from build123d import *

# Parameters (mm, degrees)
SKETCH2_R           = 19.5
SKETCH2_R_2         = 14.5
BOSS_EXTRUDE1_DEPTH = 20
BOSS_EXTRUDE2_START = 2
SKETCH3_R           = 19.5
BOSS_EXTRUDE2_DEPTH = 2
SKETCH4_R           = 2.85
BOSS_EXTRUDE3_DEPTH = 6


with BuildPart() as part:
    # Sketch2 → Boss-Extrude1 (new body)
    with BuildSketch(Plane(origin=(0, 0, 0), x_dir=(1, 0, 0), z_dir=(0, 1, 0))):
        with Locations(Location((0, 0, 0), (0, 0, 270))):
            Circle(SKETCH2_R)
        with Locations(Location((0, 0, 0), (0, 0, 270))):
            Circle(SKETCH2_R_2, mode=Mode.SUBTRACT)
    extrude(amount=BOSS_EXTRUDE1_DEPTH)

    # Sketch3 → Boss-Extrude2 (add)
    with BuildSketch(Plane.XZ.offset(BOSS_EXTRUDE2_START)):
        with Locations(Location((0, 0, 0), (0, 0, 270))):
            Circle(SKETCH3_R)
    extrude(amount=-BOSS_EXTRUDE2_DEPTH)

    # Sketch4 → Boss-Extrude3 (add)
    with BuildSketch(Plane.XZ.offset(2)):
        with Locations(Location((0, 0, 0), (0, 0, 270))):
            Circle(SKETCH4_R)
    extrude(amount=BOSS_EXTRUDE3_DEPTH)


solid = part.part
Check sheet for the modelled part. Datum: model origin and axes. Units: mm. A direction names the side the tool comes from. Coordinates: 2 decimals unless noted, no trailing zeros. Write each loop counter-clockwise with the first axis right and the second up, starting at its lowest first coordinate (ties: lowest second). Pieces come first, ordered by that corner, then holes. Notation, with made-up numbers: M 24,-25.5 L 53,-25.5 A19 cw 53,7.5 Z; hole C 26,-5.75 d7. An arc over 180 degrees is marked long. Answer as CSV lines item,"result".
Q1. Cross-section at C-C (y = 7.5). Record the boundary of the cut face in (x, z), then the cut area to 3 significant figures.
Check result:
outline,"C 0,0 d39; hole C 0,0 d29"
area,"534 mm^2"
Q2. Mould release check, pull along X, two halves, no side actions. Record for faces 1 (the face through (0, 0, 0)), 2 (the face through (-4, -2, 0)), 3 (the face through (-1.734, -4.958, 2.262)): released by +X, released by -X, zero draft, split by the parting line, or undercut.
Check result:
face 1,"undercut"
face 2,"zero draft"
face 3,"split by the parting line"
Q3. Material ranges on probe 1 along X at (y, z) = (12.5, 0); probe 2 along Y at (x, z) = (9, -14.5); probe 3 along X at (y, z) = (7.5, 2), recorded low to high. Write a range as from..to.
Check result:
probe 1,"-19.5..-14.5, 14.5..19.5"
probe 2,"-2..20"
probe 3,"-19.4..-14.36, 14.36..19.4"
Q4. Cross-section at B-B (x = -2). Record the boundary of the cut face in (y, z), then the cut area to 3 significant figures.
Check result:
outline,"M -8,-2.03 L -2,-2.03 L -2,-19.4 L 20,-19.4 L 20,-14.36 L 0,-14.36 L 0,14.36 L 20,14.36 L 20,19.4 L -2,19.4 L -2,2.03 L -8,2.03 Z"
area,"303 mm^2"
Q5. Cross-section at A-A (z = 0). Record the boundary of the cut face in (x, y), then the cut area to 3 significant figures.
Check result:
outline,"M -19.5,-2 L -2.85,-2 L -2.85,-8 L 2.85,-8 L 2.85,-2 L 19.5,-2 L 19.5,20 L 14.5,20 L 14.5,0 L -14.5,0 L -14.5,20 L -19.5,20 Z"
area,"312 mm^2"
Q6. Set-up check for faces 4 (the face through (0, -8, 0)), 5 (the face through (-5.554, 9.86, 13.394)): record each of +Z, -Z, +X, -X, +Y, -Y from which the full face is reachable in a straight line by a thin tool's end or side.
Check result:
face 4,"+Z, -Z, +X, -X, -Y"
face 5,"+Y"
Q7. Cross-section at D-D (x = 11). Record the boundary of the cut face in (y, z), then the cut area to 3 significant figures.
Check result:
outline,"M -2,-16.1 L 20,-16.1 L 20,-9.45 L 0,-9.45 L 0,9.45 L 20,9.45 L 20,16.1 L -2,16.1 Z"
area,"331 mm^2"
Q8. Go/stop test with flat-tipped pins: pin 1 (11.5 mm diameter, centred on x = 4.5, z = 8.5, fed in from -Y); pin 2 (8 mm diameter, centred on y = 9.5, z = -2, fed in from +X); pin 3 (5 mm diameter, centred on x = -6.5, y = 7.5, fed in from -Z); pin 4 (1.5 mm diameter, centred on y = -4.5, z = 12, fed in from +X). Record where each tip stops, or that it passes through.
Check result:
pin 1,"y = -2"
pin 2,"x = 19.5"
pin 3,"z = -19.09"
pin 4,"through"
